Geometry check sheet. Reference: the model listing, model coordinates, mm. A direction names the side the tool comes from. Give positions to 0.01 mm unless a question says otherwise; leave off trailing zeros. Order: outer loops, then holes, each group sorted by start corner. A loop starts at its lowest first (then second) coordinate and runs counter-clockwise, first axis right, second up. Notation, with made-up numbers: M 25.25,9.25 L 49.25,9.25 A11 cw 49.25,27.25 Z; hole C -4.5,18 d1. An arc over 180 degrees is marked long. Put each result on its own line as item: value. Start each with the question number.
Q1. Material ranges on L1, parallel to X at y = 6, z = 5.5; L2, parallel to Y at x = -1.5, z = 17.5; L3, parallel to Z at x = 1, y = 6.75, recorded low to high.
Q2. Access from +Z, -Z, +X, -X, +Y, -Y to the whole of each face (thin tool, end or side, straight path). Record for faces 4 (the flat face through (4.724, 1, 16)), 5 (the flat face through (3.24, 0.99, -4.72)), 6 (the flat face through (0, 2, -11)), 7 (the flat face through (-3.791, 0.986, 12.167)), 8 (the flat face through (-3.791, 0.986, -11.833)).
Q3. Go/stop test with flat-tipped pins: pin 1 (4 mm diameter, centred on y = 6, z = 4.5, fed in from +X); pin 2 (3 mm diameter, centred on x = 3, z = 16, fed in from -Y); pin 3 (3 mm diameter, centred on y = 7.5, z = 0.5, fed in from -X); pin 4 (4 mm diameter, centred on x = -0.28, z = 15.72, fed in from +Y). Record where each tip stops, or that it passes through.
Q4. Mould release check, pull along Y, two halves, no side actions. Record for faces 1 (the flat face through (0, 2, 13)), 2 (the cylindrical face through (-0.247, 4.536, 4.048)), 3 (the flat face through (0, 4, -3.277)): +Y half, -Y half, draft (parallel to the pull), parting line (faces both ways), or undercut.
Q5. Section check B-B on z = -8. Record the cut outline in (x, y), then the cut area to 3 significant figures.
Q6. Section check D-D on y = 1. Record the cut outline in (x, z), then the cut area to 3 significant figures.
Q7. Section check A-A on x = 2.5. Record the cut outline in (y, z), then the cut area to 3 significant figures.
Q8. Section check C-C on x = 0.5. Record the cut outline in (y, z).
```python
from build123d import *

# Parameters (mm, degrees)
BOSS_EXTRU_1_DEPTH             = 2
BOSS_EXTRU_2_REACH             = 23.477
BOSS_EXTRU_2_DIRECTION_2_REACH = 23.477
ESQUISSE6_R                    = 1.5
ENL_V_MAT_EXTRU_3_DEPTH        = 26.464516662
ESQUISSE7_R                    = 1.75
ENL_V_MAT_EXTRU_4_DEPTH        = 25.047357729


with BuildPart() as part:
    # Esquisse1 → Boss.-Extru.1 (new body)
    with BuildSketch(Plane(origin=(0, 0, 0), x_dir=(1, 0, 0), z_dir=(0, 1, 0))):
        Polygon((1.795292522, 13.277027027), (-2.346843102, 13.277027027), (-5.27577529, 10.348094839), (-5.27577529, 6.205959215), (-2.346843102, 3.277027027), (-2.346843102, -10.722972973), (-5.27577529, -13.651905161), (-5.27577529, -17.794040785), (-2.346843102, -20.722972973), (1.795292522, -20.722972973), (4.72422471, -17.794040785), (4.72422471, -13.651905161), (1.795292522, -10.722972973), (1.795292522, 3.277027027), (4.72422471, 6.205959215), (4.72422471, 10.348094839), align=None)
    extrude(amount=BOSS_EXTRU_1_DEPTH)

    # Boss.-Extru.2: up to this face of the body (flat: up to its plane)
    boss_extru_2_end = Plane(part.part.faces().sort_by_distance((1.795292522, 1, 3.722972973))[0])
    # Esquisse3 → Boss.-Extru.2 (add, up to the picked face)
    with BuildSketch(Plane(origin=(0, 0, 0), x_dir=(0, 0, -1), z_dir=(1, 0, 0)), mode=Mode.PRIVATE) as boss_extru_2_sk1:
        with BuildLine():
            Line((-10.722972973, 0), (-10.722972973, 6))
            ThreePointArc((-10.722972973, 6), (-3.722972973, 13), (3.277027027, 6))
            Line((3.277027027, 6), (3.277027027, 0))
            Line((3.277027027, 0), (-10.722972973, 0))
        make_face()
    boss_extru_2_tool1 = split(extrude(boss_extru_2_sk1.sketch, amount=BOSS_EXTRU_2_REACH, mode=Mode.PRIVATE), bisect_by=boss_extru_2_end, keep=Keep.BOTH, mode=Mode.PRIVATE)
    add(boss_extru_2_tool1.solids().sort_by(Axis((0, 5.855045, 3.722973), (1, 0, 0)))[0])

    # Boss.-Extru.2 direction 2: up to this face of the body (flat: up to its plane)
    boss_extru_2_direction_2_end = Plane(part.part.faces().sort_by_distance((-2.346843102, 1, 3.722972973))[0])
    # Esquisse3 → Boss.-Extru.2 direction 2 (add, up to the picked face)
    with BuildSketch(Plane(origin=(0, 0, 0), x_dir=(0, 0, -1), z_dir=(1, 0, 0)), mode=Mode.PRIVATE) as boss_extru_2_direction_2_sk1:
        with BuildLine():
            Line((-10.722972973, 0), (-10.722972973, 6))
            ThreePointArc((-10.722972973, 6), (-3.722972973, 13), (3.277027027, 6))
            Line((3.277027027, 6), (3.277027027, 0))
            Line((3.277027027, 0), (-10.722972973, 0))
        make_face()
    boss_extru_2_direction_2_tool1 = split(extrude(boss_extru_2_direction_2_sk1.sketch, amount=-BOSS_EXTRU_2_DIRECTION_2_REACH, mode=Mode.PRIVATE), bisect_by=boss_extru_2_direction_2_end, keep=Keep.BOTH, mode=Mode.PRIVATE)
    add(boss_extru_2_direction_2_tool1.solids().sort_by(Axis((0, 5.855045, 3.722973), (-1, 0, 0)))[0])

    # Esquisse6 → Enlèv. mat.-Extru.3 (cut, through all)
    with BuildSketch(Plane(origin=(1.795292522, 0, 0), x_dir=(0, 0, -1), z_dir=(1, 0, 0))):
        with Locations((-3.722972973, 6)):
            Circle(ESQUISSE6_R)
    extrude(amount=-ENL_V_MAT_EXTRU_3_DEPTH, mode=Mode.SUBTRACT)

    # Esquisse7 → Enlèv. mat.-Extru.4 (cut, through all)
    with BuildSketch(Plane(origin=(0, 2, 0), x_dir=(1, 0, 0), z_dir=(0, 1, 0))):
        with Locations(Location((-0.27577529, -15.722972973, 0), (0, 0, 270))):
            Circle(ESQUISSE7_R)
        with Locations(Location((-0.27577529, 8.277027027, 0), (0, 0, 270))):
            Circle(ESQUISSE7_R)
    extrude(amount=-ENL_V_MAT_EXTRU_4_DEPTH, mode=Mode.SUBTRACT)


solid = part.part
```
Results found:
1. L1: x = -2.35 to 1.8
1. L2: y = 0 to 2
1. L3: z = -3.24 to 2.42, 5.02 to 10.68
2. face 4: +Z, -Z, +X, +Y, -Y
2. face 5: +X, +Y, -Y
2. face 6: -Z, +X, -X, +Y
2. face 7: -X, +Y, -Y
2. face 8: -Z, -X, +Y, -Y
3. pin 1: stops at x = 1.8
3. pin 2: stops at y = 0
3. pin 3: stops at x = -2.35
3. pin 4: stops at y = 2
4. face 1: +Y half
4. face 2: undercut
4. face 3: draft
5. outline: M -5.28,0 L -2,0 L -2,2 L -5.28,2 Z; M 1.45,0 L 4.72,0 L 4.72,2 L 1.45,2 Z
5. area: 13.1 mm^2
6. outline: M -5.28,-10.35 L -2.35,-13.28 L 1.8,-13.28 L 4.72,-10.35 L 4.72,-6.21 L 1.8,-3.28 L 1.8,10.72 L 4.72,13.65 L 4.72,17.79 L 1.8,20.72 L -2.35,20.72 L -5.28,17.79 L -5.28,13.65 L -2.35,10.72 L -2.35,-3.28 L -5.28,-6.21 Z; hole C -0.28,-8.28 d3.5; hole C -0.28,15.72 d3.5
6. area: 204 mm^2
7. outline: M 0,-12.57 L 2,-12.57 L 2,-3.98 L 0,-3.98 Z; M 0,11.43 L 2,11.43 L 2,20.02 L 0,20.02 Z
7. area: 34.4 mm^2
8. outline: M 0,-13.28 L 2,-13.28 L 2,-9.85 L 0,-9.85 Z; M 0,-6.71 L 2,-6.71 L 2,-3.28 L 6,-3.28 A7 ccw 6,10.72 L 2,10.72 L 2,14.15 L 0,14.15 Z; M 0,17.29 L 2,17.29 L 2,20.72 L 0,20.72 Z; hole C 6,3.72 d3
